Job drawing, mm, ordinate dimensions from the low corner. One solid piece. Give positions to 0.01 mm unless a question says otherwise; leave off trailing zeros. Loops run counter-clockwise (first coordinate to the right, second up) from the corner with the lowest first, then second, coordinate; pieces in that order, holes last.
Item 1: Saw through at A-A on y = 80.5. Give the cut face in (x, z).
Item 2: Drop flat-ended pins along their axis: P1, Ø1.5, axis at x = 27, z = 3.5, coming from the +Y side; P2, Ø1.8, axis at y = 306.5, z = 2, coming from the -X side; P3, Ø2, axis at x = 14, z = 10.5, coming from the +Y side. Give the stop position or say it passes through.
Item 3: Probe probe 1 along X at (y, z) = (137, 5); probe 2 along Z at (x, y) = (4.5, 96); probe 3 along Y at (x, z) = (7.5, 11.75). List the from-to ranges inside material, lowest first.
Item 4: Saw through at C-C on z = 2.25. Give the cut face in (x, y).
Item 5: Saw through at B-B on x = 14. Give the cut face in (y, z).
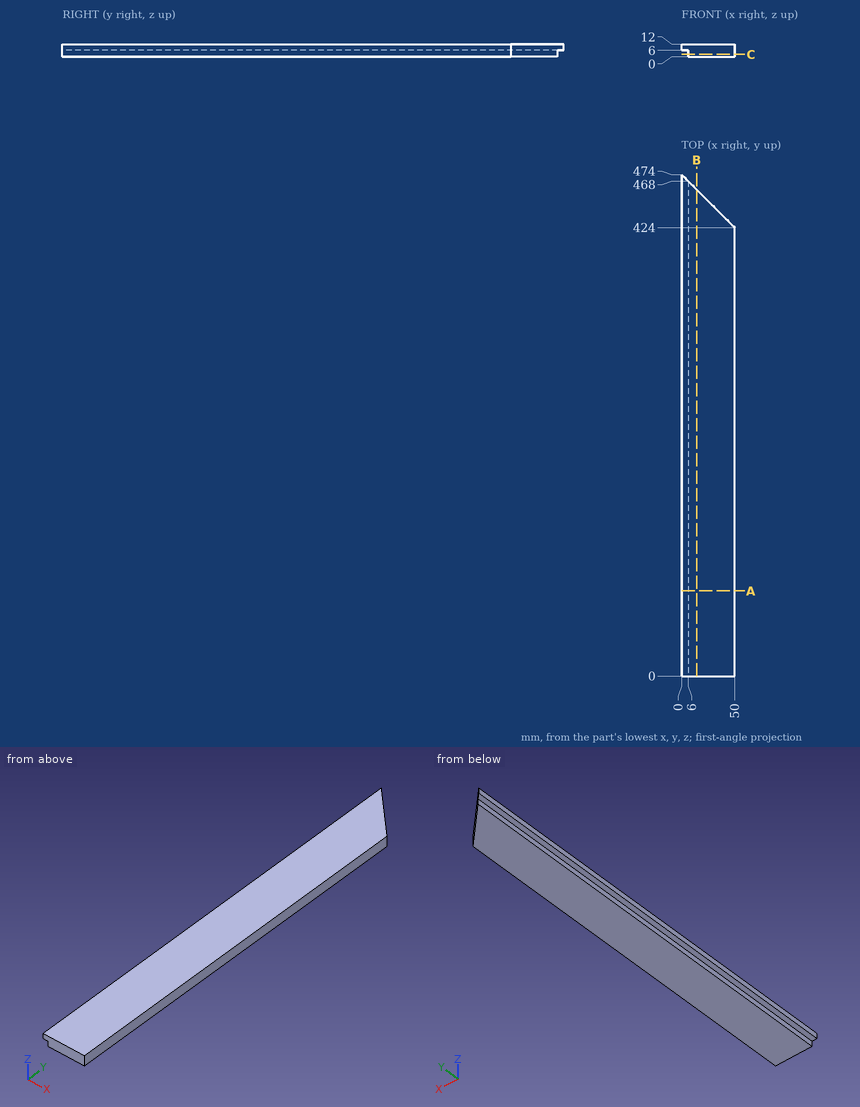
Results below:
1. outline: (0, 6) - (6, 6) - (6, 0) - (50, 0) - (50, 12) - (0, 12) - close
2. P1: stops at y = 447.75
2. P2: stops at x = 6
2. P3: stops at y = 461
3. probe 1: x = 6 to 50
3. probe 2: z = 6 to 12
3. probe 3: y = 0 to 466.5
4. outline: (6, 0) - (50, 0) - (50, 424) - (6, 468) - close
5. outline: (0, 0) - (460, 0) - (460, 12) - (0, 12) - close
